```python
from build123d import *

# Parameters (mm, degrees)
SKETCH1_R           = 50.8
BOSS_EXTRUDE1_DEPTH = 19.05
CUT_EXTRUDE2_DEPTH  = 15.24
SKETCH5_R           = 4.064
CUT_EXTRUDE3_DEPTH  = 74.440708058
CUT_EXTRUDE4_DEPTH  = 75.324844433
SKETCH7_R           = 48.26
GUTTED_DEPTH        = 15.24


with BuildPart() as part:
    # Sketch1 → Boss-Extrude1 (new body)
    with BuildSketch(Plane(origin=(0, 0, 0), x_dir=(1, 0, 0), z_dir=(0, 1, 0))):
        with Locations(Location((0, 0, 0), (0, 0, 90))):
            Circle(SKETCH1_R)
    extrude(amount=BOSS_EXTRUDE1_DEPTH)

    # Sketch4 → Cut-Extrude2 (cut)
    with BuildSketch(Plane(origin=(0, 19.05, 0), x_dir=(1, 0, 0), z_dir=(0, 1, 0))):
        Polygon((-3.519527241, 6.096), (3.519527241, 6.096), (7.039054482, 0), (3.519527241, -6.096), (-3.519527241, -6.096), (-7.039054482, 0), align=None)
    extrude(amount=-CUT_EXTRUDE2_DEPTH, mode=Mode.SUBTRACT)

    # Sketch5 → Cut-Extrude3 (cut, through all)
    with BuildSketch(Plane(origin=(0, 3.81, 0), x_dir=(1, 0, 0), z_dir=(0, 1, 0))):
        with Locations(Location((0, 0, 0), (0, 0, 270))):
            Circle(SKETCH5_R)
    extrude(amount=-CUT_EXTRUDE3_DEPTH, mode=Mode.SUBTRACT)

    # Sketch6 → Cut-Extrude4 (cut, through all)
    with BuildSketch(Plane(origin=(0, 19.05, 0), x_dir=(1, 0, 0), z_dir=(0, 1, 0))):
        with BuildLine():
            ThreePointArc((-13.470384182, 13.470384182), (-7.290119387, 17.599905094), (0, 19.05))
            Line((0, 19.05), (0, 38.1))
            ThreePointArc((0, 38.1), (-14.580238773, 35.199810189), (-26.940768363, 26.940768363))
            Line((-26.940768363, 26.940768363), (-13.470384182, 13.470384182))
        make_face()
        with BuildLine():
            Line((26.940768363, 26.940768363), (13.470384182, 13.470384182))
            ThreePointArc((13.470384182, 13.470384182), (17.599905094, 7.290119387), (19.05, 0))
            Line((19.05, 0), (38.1, 0))
            ThreePointArc((38.1, 0), (35.199810189, 14.580238773), (26.940768363, 26.940768363))
        make_face()
        with BuildLine():
            Line((26.940768363, -26.940768363), (13.470384182, -13.470384182))
            ThreePointArc((13.470384182, -13.470384182), (7.290119387, -17.599905094), (0, -19.05))
            Line((0, -19.05), (0, -38.1))
            ThreePointArc((0, -38.1), (14.580238773, -35.199810189), (26.940768363, -26.940768363))
        make_face()
        with BuildLine():
            Line((-26.940768363, -26.940768363), (-13.470384182, -13.470384182))
            ThreePointArc((-13.470384182, -13.470384182), (-17.599905094, -7.290119387), (-19.05, 0))
            Line((-19.05, 0), (-38.1, 0))
            ThreePointArc((-38.1, 0), (-35.199810189, -14.580238773), (-26.940768363, -26.940768363))
        make_face()
    extrude(amount=-CUT_EXTRUDE4_DEPTH, mode=Mode.SUBTRACT)

    # Sketch7 → gutted (cut)
    with BuildSketch(Plane(origin=(0, 19.05, 0), x_dir=(1, 0, 0), z_dir=(0, 1, 0))):
        with Locations(Location((0, 0, 0), (0, 0, 270))):
            Circle(SKETCH7_R)
        with BuildLine():
            Line((-16.313445375, 2.54), (-40.560547334, 2.54))
            ThreePointArc((-40.560547334, 2.54), (-37.546464201, -15.552254691), (-26.884586844, -30.476689292))
            Line((-26.884586844, -30.476689292), (-9.739296625, -13.331399073))
            ThreePointArc((-9.739296625, -13.331399073), (-15.253251082, -6.318103468), (-16.313445375, 2.54))
        make_face(mode=Mode.SUBTRACT)
        with BuildLine():
            Line((16.313445375, -2.54), (40.560547334, -2.54))
            ThreePointArc((40.560547334, -2.54), (37.546464201, 15.552254691), (26.884586844, 30.476689292))
            Line((26.884586844, 30.476689292), (9.739296625, 13.331399073))
            ThreePointArc((9.739296625, 13.331399073), (15.253251082, 6.318103468), (16.313445375, -2.54))
        make_face(mode=Mode.SUBTRACT)
        Polygon((4.985996925, 8.636), (-4.985996925, 8.636), (-9.971993849, 0), (-4.985996925, -8.636), (4.985996925, -8.636), (9.971993849, 0), align=None, mode=Mode.SUBTRACT)
        with BuildLine():
            ThreePointArc((2.54, 40.560547334), (-15.552254691, 37.546464201), (-30.476689292, 26.884586844))
            Line((-30.476689292, 26.884586844), (-13.331399073, 9.739296625))
            ThreePointArc((-13.331399073, 9.739296625), (-6.318103468, 15.253251082), (2.54, 16.313445375))
            Line((2.54, 16.313445375), (2.54, 40.560547334))
        make_face(mode=Mode.SUBTRACT)
        with BuildLine():
            Line((-2.54, -16.313445375), (-2.54, -40.560547334))
            ThreePointArc((-2.54, -40.560547334), (15.552254691, -37.546464201), (30.476689292, -26.884586844))
            Line((30.476689292, -26.884586844), (13.331399073, -9.739296625))
            ThreePointArc((13.331399073, -9.739296625), (6.318103468, -15.253251082), (-2.54, -16.313445375))
        make_face(mode=Mode.SUBTRACT)
    extrude(amount=-GUTTED_DEPTH, mode=Mode.SUBTRACT)


solid = part.part
```
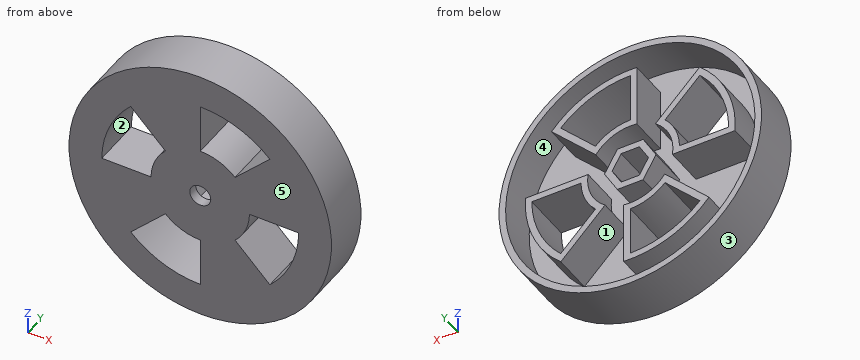
Input: part model. Units: mm. Frame: model coordinates. Face numbers are marked on the shaded views. A direction names the side the tool comes from. Coordinates: 2 decimals unless noted, no trailing zeros. Loops run counter-clockwise (first coordinate to the right, second up) from the corner with the lowest first, then second, coordinate; pieces in that order, holes last. Notation, with made-up numbers: (76, 75.5) - (123, 75.5) arc R23 ccw to (123, 84.5) - close; hole circle Ø3 at (8.25, 81). An arc over 180 degrees is marked (long way). Answer in a Markdown table with one row per item.
(1) Cut plane A-A on z = 32.5. Output: boundary loops of the cut face in (x, y).
Model answer:
| item | result |
|---|---|
| outline | (-39.04, 0) - (0, 0) - (0, 19.05) - (-2.54, 19.05) - (-2.54, 3.81) - (-35.68, 3.81) - (-35.68, 19.05) - (-39.04, 19.05) - close; (19.88, 0) - (39.04, 0) - (39.04, 19.05) - (35.68, 19.05) - (35.68, 3.81) - (24.4, 3.81) - (24.4, 19.05) - (19.88, 19.05) - close |
(2) Pin query (flat end, axial travel): P1, Ø3, axis at x = -11.5, z = 21.5, coming from the -Y side; P2, Ø9.5, axis at y = 9, z = -26, coming from the -X side; P3, Ø7.5, axis at y = 15, z = -31, coming from the +X side; P4, Ø4, axis at y = 11.5, z = -23.5, coming from the +X side. Return the tip coordinate at first contact, or that it passes through.
Model answer:
| item | result |
|---|---|
| P1 | stops at y = 0 |
| P2 | stops at x = -46.14 |
| P3 | stops at x = 42.87 |
| P4 | stops at x = 46.03 |
(3) Cut plane B-B on y = 7.25. Count the separate pieces of the cut face and the enclosed holes in it, plus the area to 3 significant figures.
Model answer:
| item | result |
|---|---|
| separate pieces | 6 |
| enclosed holes | 6 |
| area | 1,870 mm² |
(4) Material intervals for L1, parallel to Z at x = 34.5, y = 10.75; L2, parallel to X at y = 9, z = 17; L3, parallel to X at y = 6.75, z = 33, sorted ascending. Write a range as from..to.
Model answer:
| item | result |
|---|---|
| L1 | z = -37.29..-33.75, -21.48..-16.17, 0..2.54, 33.75..37.29 |
| L2 | x = -47.87..-45.17, -36.91..-34.1, -17..-13.41, -2.54..8.6, 17..20.59, 45.17..47.87 |
| L3 | x = -38.62..-35.21, -2.54..0, 19.04..23.72, 35.21..38.62 |
(5) Cut plane C-C on x = -33.5. Output: boundary loops of the cut face in (y, z).
Model answer:
| item | result |
|---|---|
| outline | (0, -38.19) - (19.05, -38.19) - (19.05, -34.74) - (3.81, -34.74) - (3.81, -2.54) - (19.05, -2.54) - (19.05, 0) - (0, 0) - close; (0, 18.15) - (19.05, 18.15) - (19.05, 23.01) - (3.81, 23.01) - (3.81, 34.74) - (19.05, 34.74) - (19.05, 38.19) - (0, 38.19) - close |
(6) Set-up query: the marked faces 1 and 2. Return all of +Z, -Z, +X, -X, +Y, -Y with unobstructed straight access to the full face (end or side cutting, diameter ignored); none if empty.
Model answer:
| item | result |
|---|---|
| face 1 | +Y |
| face 2 | +Y, -Y |
(7) Mould query, pull axis X, two halves, no side actions, for the marked faces 3, 4 and 5. Classes: pulls with the +X half, pulls with the -X half, needs draft (parallel to the pull), parting line crosses it, or undercut.
Model answer:
| item | result |
|---|---|
| face 3 | parting line crosses it |
| face 4 | undercut |
| face 5 | needs draft |
